from build123d import *

# Parameters (mm, degrees)
EXTRUDE1_DEPTH = 30
FILLET1_R      = 1


with BuildPart() as part:
    # Sketch1 → Extrude1 (new body)
    with BuildSketch(Plane.XY):
        Polygon((0, 0), (-30, 0), (-30, -3), (-3, -3), (-3, -30), (0, -30), align=None)
    extrude(amount=EXTRUDE1_DEPTH)

    # Fillet1
    fillet1_edges = [part.edges().sort_by_distance(p)[0] for p in [
        (-3, -30, 15),
        (-3, -3, 15),
        (-30, -3, 15),
    ]]
    fillet(fillet1_edges, radius=FILLET1_R)


solid = part.part
Could you check a few things on this model? Use its own coordinates, in mm. A direction names the side the tool comes from. Give positions to 0.01 mm unless a question says otherwise; leave off trailing zeros. Loops run counter-clockwise (first coordinate to the right, second up) from the corner with the lowest first, then second, coordinate; pieces in that order, holes last. Notation, with made-up numbers: M 75.25,5 L 106.25,5 A27 ccw 106.25,42 Z; hole C 16.5,21 d5. An arc over 180 degrees is marked long. Answer as a JSON object with one key per item and string values.
Q1. If I drill on probe 1 along X at (y, z) = (-10, 23), over which ranges is the centre line in solid material (lowest first)? Write a range as [from, to].
Values found:
{"probe 1": "x = [-3, 0]"}
Q2. Suppose I cut it at B-B, the plane x = -7.5. List the corners of the cut face in (y, z) for me.
Values found:
{"outline": "M -3,0 L 0,0 L 0,30 L -3,30 Z"}
Q3. Suppose I cut it at A-A, the plane z = 9. List the corners of the cut face in (x, y) for me, plus the area to 3 significant figures.
Values found:
{"outline": "M -30,-2 A1 ccw -29,-3 L -4,-3 A1 cw -3,-4 L -3,-29 A1 ccw -2,-30 L 0,-30 L 0,0 L -30,0 Z", "area": "171 mm²"}
Q4. For faces 1 (the flat face through (-17, -3, 15)), 2 (the flat face through (-15, 0, 15)), which set-ups out of +Z, -Z, +X, -X, +Y, -Y let a thin tool reach every point of the face, with its end or its side?
Values found:
{"face 1": "+Z, -Z, -X, -Y", "face 2": "+Z, -Z, +X, -X, +Y"}
Q5. For P1, Ø1, axis at y = -16.5, z = 11.5, coming from the -X side; P2, Ø3, axis at x = -20, z = 5, coming from the -Y side; P3, Ø1.5, axis at y = -3.5, z = 18.5, coming from the -X side, each with a flat end and sliding along its axis, tell me the tip position at first contact or that it passes through.
Values found:
{"P1": "stops at x = -3", "P2": "stops at y = -3", "P3": "stops at x = -29.66"}
